Source: CAD feature listing. Evaluate the final solid. Frame: model axes, mm. A direction names the side the tool comes from. Give positions to 0.01 mm unless a question says otherwise; leave off trailing zeros. Answer as a JSON object with one key per item and string values. Group by question number.
from build123d import *

# Parameters (mm, degrees)
SKETCH1_R                   = 88.9
BASE_DEPTH                  = 12.7
SKETCH1_4_R                 = 114.3
SKETCH1_4_R_2               = 88.9
BOLT_BELT_DEPTH             = 12.7
F_3_8_24_TAPPED_HOLE1_D     = 8.4328
SKETCH21_R                  = 82.55
ENGINE_OFFSET_DEPTH         = 12.7
SKETCH20_W                  = 165.1
SKETCH20_H                  = 215.9
ENGINE_BLOCK_DEPTH          = 63.5
ENGINE_BLOCK_FILLET_FRONT_R = 25.4
ENGINE_BLOCK_FILLET_BACK_R  = 12.7
SKETCH22_W                  = 6.35
SKETCH22_H                  = 25.4
FINS_DEPTH                  = 63.5
FIN_LPATTERN1_COUNT         = 4
FIN_LPATTERN1_PITCH         = 12.7
FIN_LPATTERN1_COL_COUNT     = 4
FIN_LPATTERN1_COL_PITCH     = 12.7
SHROUD_DEPTH                = 38.1
SHROUD_TAPER                = 15
SKETCH24_R                  = 50.8
CORD_HOUSING_DEPTH          = 31.75
CORD_HOUSING_TAPER          = 10
CORD_HOUSING_FILLET_R       = 12.7
SKETCH25_R                  = 9.525
BOSS_EXTRUDE7_DEPTH         = 25.4


with BuildPart() as part:
    # Sketch1 → Base (new body)
    with BuildSketch(Plane(origin=(0, 0, 0), x_dir=(1, 0, 0), z_dir=(0, 1, 0))):
        with Locations(Location((0, 0, 0), (0, 0, 270))):  # turned: the seam where the file's is
            Circle(SKETCH1_R)
    extrude(amount=-BASE_DEPTH)

    # Sketch1_4 → Bolt Belt (add)
    with BuildSketch(Plane(origin=(0, 0, 0), x_dir=(1, 0, 0), z_dir=(0, 1, 0))):
        with Locations(Location((0, 0, 0), (0, 0, 270))):  # turned: the seam where the file's is
            Circle(SKETCH1_4_R)
        with Locations(Location((0, 0, 0), (0, 0, 270))):  # turned: the seam where the file's is
            Circle(SKETCH1_4_R_2, mode=Mode.SUBTRACT)
        with Locations(Location((0, 0, 0), (0, 0, 270))):  # turned: the seam where the file's is
            Circle(SKETCH1_4_R_2)
    extrude(amount=BOLT_BELT_DEPTH)

    # 3_8-24 Tapped Hole1 (through all)
    with Locations(Plane.XZ):
        with Locations((-70.63929059, 73.025), (89.644179842, 47.817162405), (-55.633966752, -85.014244356)):
            Hole(F_3_8_24_TAPPED_HOLE1_D / 2)

    # Sketch21 → Engine Offset (add)
    with BuildSketch(Plane(origin=(0, 12.7, 0), x_dir=(1, 0, 0), z_dir=(0, 1, 0))):
        with Locations(Location((0, 0, 0), (0, 0, 270))):  # turned: the seam where the file's is
            Circle(SKETCH21_R)
    extrude(amount=ENGINE_OFFSET_DEPTH)

    # Sketch20 → Engine Block (add)
    with BuildSketch(Plane(origin=(0, 25.4, 0), x_dir=(1, 0, 0), z_dir=(0, 1, 0))):
        with Locations((0, 6.35)):
            Rectangle(SKETCH20_W, SKETCH20_H)
    extrude(amount=ENGINE_BLOCK_DEPTH)

    # Engine Block Fillet Front
    engine_block_fillet_front_edges = [part.edges().sort_by_distance(p)[0] for p in [
        (-82.55, 57.15, 101.6),
        (82.55, 57.15, 101.6),
    ]]
    fillet(engine_block_fillet_front_edges, radius=ENGINE_BLOCK_FILLET_FRONT_R)

    # Engine Block Fillet Back
    engine_block_fillet_back_edges = [part.edges().sort_by_distance(p)[0] for p in [
        (-82.55, 57.15, -114.3),
        (82.55, 57.15, -114.3),
    ]]
    fillet(engine_block_fillet_back_edges, radius=ENGINE_BLOCK_FILLET_BACK_R)

    # Sketch22 → Fins (cut)
    with BuildSketch(Plane(origin=(0, 88.9, 0), x_dir=(1, 0, 0), z_dir=(0, 1, 0))):
        with Locations((0, -101.6)):
            Rectangle(SKETCH22_W, SKETCH22_H)
    fins = extrude(amount=-FINS_DEPTH, mode=Mode.SUBTRACT)

    # Fin LPattern1: Fins ×4
    with Locations(*[(i * FIN_LPATTERN1_PITCH, 0, 0) for i in range(1, FIN_LPATTERN1_COUNT)]):
        add(fins, mode=Mode.SUBTRACT)

    # Fin LPattern1 col: Fins ×4
    with Locations(*[(-i * FIN_LPATTERN1_COL_PITCH, 0, 0) for i in range(1, FIN_LPATTERN1_COL_COUNT)]):
        add(fins, mode=Mode.SUBTRACT)

    # Sketch23 → Shroud (add)
    with BuildSketch(Plane(origin=(0, 88.9, 0), x_dir=(1, 0, 0), z_dir=(0, 1, 0))):
        with BuildLine():
            ThreePointArc((82.55, 31.75), (0, 114.3), (-82.55, 31.75))
            Line((-82.55, 31.75), (-82.55, -88.9))
            ThreePointArc((-82.55, -88.9), (-67.671024484, -124.821024484), (-31.75, -139.7))
            Line((-31.75, -139.7), (31.75, -139.7))
            ThreePointArc((31.75, -139.7), (67.671024484, -124.821024484), (82.55, -88.9))
            Line((82.55, -88.9), (82.55, 31.75))
        make_face()
    extrude(amount=SHROUD_DEPTH, taper=SHROUD_TAPER)

    # Sketch24 → Cord Housing (add)
    with BuildSketch(Plane(origin=(0, 127, 0), x_dir=(1, 0, 0), z_dir=(0, 1, 0))):
        with Locations((0, 31.75)):
            Circle(SKETCH24_R)
    extrude(amount=CORD_HOUSING_DEPTH, taper=CORD_HOUSING_TAPER)

    # Cord Housing Fillet
    cord_housing_fillet_edges = [part.edges().sort_by_distance(p)[0] for p in [
        (-45.201618363, 158.75, -31.75),
    ]]
    fillet(cord_housing_fillet_edges, radius=CORD_HOUSING_FILLET_R)

    # Sketch25 → Boss-Extrude7 (add)
    with BuildSketch(Plane.XZ.offset(12.7)):
        with Locations(Location((0, 0, 0), (0, 0, 90))):  # turned: the seam where the file's is
            Circle(SKETCH25_R)
    extrude(amount=BOSS_EXTRUDE7_DEPTH)


solid = part.part
Q1. First-contact query: pin 1 Ø6.5 at (y, z) = (44, 92.5) entering from -X; pin 2 Ø1.5 at (y, z) = (123.5, -42.5) entering from -X; pin 3 Ø4 at (y, z) = (50, 97.5) entering from +X. Flat tips, straight axial feed; report the tip coordinate or a pass-through.
Q2. Reachability of faces 1 (the flat face through (-15.875, 58, 95)), 2 (the cylindrical face through (-74.66, 6.44, 74.29)), 3 (the conical face through (-6.149, 147.223, -78.582)), 4 (the flat face through (32, 57, 101.6)) from +Z, -Z, +X, -X, +Y, -Y: full face, straight path, thin tool, end or side. Return the list, or none.
Q3. Draft query along X for faces 5 (the cylindrical face through (78.73, 57.59, -110.68)), 6 (the conical face through (-64.364, 108.217, 120.804)), 7 (the flat face through (-3.175, 58, 95)), 8 (the flat face through (0, 158.75, -32)). Return one class per face: released by +X, released by -X, zero draft, split by the parting line, or undercut.
Q4. Ray query, probe 1 along Y at (x, z) = (21.5, 89.5); probe 2 along X at (y, z) = (31, -88.5); probe 3 along Z at (x, y) = (-47.5, 26.5). Return the intervals inside material, ascending. Write a range as [from, to].
Taken from the geometry:
{
 "1": {"pin 1": "stops at x = -78.94", "pin 2": "stops at x = -72.72", "pin 3": "stops at x = 73.66"},
 "2": {"face 1": "+Z", "face 2": "-Y", "face 3": "+Y", "face 4": "+Z, +X, -X"},
 "3": {"face 5": "released by +X", "face 6": "released by -X", "face 7": "undercut", "face 8": "zero draft"},
 "4": {"probe 1": "y = [0, 12.7], [25.4, 127]", "probe 2": "x = [-82.55, 82.55]", "probe 3": "z = [-114.3, 101.6]"}
}
